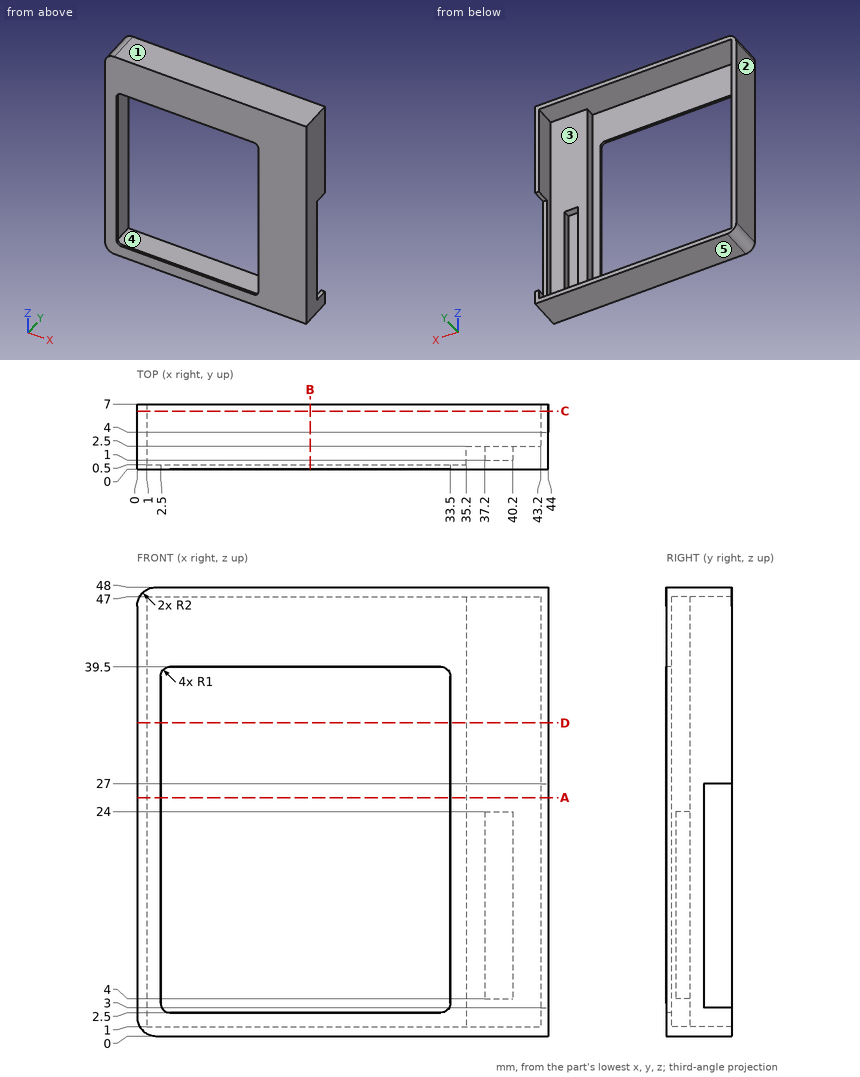
Could you check a few things on this drawing? It's one solid part, dimensions in mm from its lowest x, y, z. A direction names the side the tool comes from. Round coordinates to 2 decimals unless told otherwise and drop trailing zeros. Order: outer loops, then holes, each group sorted by start corner. A loop starts at its lowest first (then second) coordinate and runs counter-clockwise, first axis right, second up.
Q1. Imagine slicing it at B-B, the plane x = 18.5. List the corners of the cut face in (y, z) for me.
Geometry says:
outline: (0, 0) - (7, 0) - (7, 1) - (0.5, 1) - (0.5, 2.5) - (0, 2.5) - close; (0, 39.5) - (0.5, 39.5) - (0.5, 47) - (7, 47) - (7, 48) - (0, 48) - close
Q2. Please list where these lines run through material, in increasing order: probe 1 along X at (y, z) = (1.75, 12); probe 2 along Z at (x, y) = (28.5, 2.25); probe 3 along X at (y, z) = (5, 37).
Geometry says:
probe 1: x = 0 to 1, 35.2 to 37.2, 40.2 to 44
probe 2: z = 0 to 1, 47 to 48
probe 3: x = 0 to 1, 43.2 to 44
Q3. Imagine slicing it at C-C, the plane y = 6.25. List the corners of the cut face in (x, z) for me.
Geometry says:
outline: (0, 2) arc R2 ccw to (2, 0) - (44, 0) - (44, 3) - (43.2, 3) - (43.2, 1) - (1, 1) - (1, 47) - (43.2, 47) - (43.2, 27) - (44, 27) - (44, 48) - (2, 48) arc R2 ccw to (0, 46) - close
Q4. I'm going to push flat-ended pins straight in: P1, Ø10.5, axis at x = 26, z = 15.5, coming from the +Y side; P2, Ø6.5, axis at x = 38.5, z = 29, coming from the +Y side. Where does each tip first touch, or does it pass through?
Geometry says:
P1: passes through
P2: stops at y = 2.5
Q5. Which directions (+Z, -Z, +X, -X, +Y, -Y) give clear straight access to the entire face, cutting with the end or side of a thin tool? Please do the marked faces 4 and 5.
Geometry says:
face 4: +Y
face 5: -Z, +X, -X, +Y, -Y
Q6. Thinking about a two-plate mould opening in X: for the marked faces 1, 2 and 3, which applies, released by +X, released by -X, zero draft, split by the parting line, or undercut?
Geometry says:
face 1: zero draft
face 2: released by -X
face 3: undercut
Q7. Imagine slicing it at A-A, the plane z = 25.5. List the corners of the cut face in (x, y) for me, then the cut area to 3 significant figures.
Geometry says:
outline: (0, 0) - (2.5, 0) - (2.5, 0.5) - (1, 0.5) - (1, 7) - (0, 7) - close; (33.5, 0) - (44, 0) - (44, 4) - (43.2, 4) - (43.2, 2.5) - (35.2, 2.5) - (35.2, 0.5) - (33.5, 0.5) - close
area: 31.8 mm2
Q8. Imagine slicing it at D-D, the plane z = 33.5. List the corners of the cut face in (x, y) for me, then the cut area to 3 significant figures.
Geometry says:
outline: (0, 0) - (2.5, 0) - (2.5, 0.5) - (1, 0.5) - (1, 7) - (0, 7) - close; (33.5, 0) - (44, 0) - (44, 7) - (43.2, 7) - (43.2, 2.5) - (35.2, 2.5) - (35.2, 0.5) - (33.5, 0.5) - close
area: 34.2 mm2
